Study the drawing (mm; zero at the part's minimum x, y, z) and answer. Round coordinates to 2 decimals unless told otherwise and drop trailing zeros. Loops run counter-clockwise (first coordinate to the right, second up) from the corner with the lowest first, then second, coordinate; pieces in that order, holes last. Notation, with made-up numbers: M -27,-14 L 6,-14 A13 cw 6,-10 Z; hole C -1,-32 d7. An arc over 180 degrees is marked long. Write each question's results on one line, items separated by ' | '.
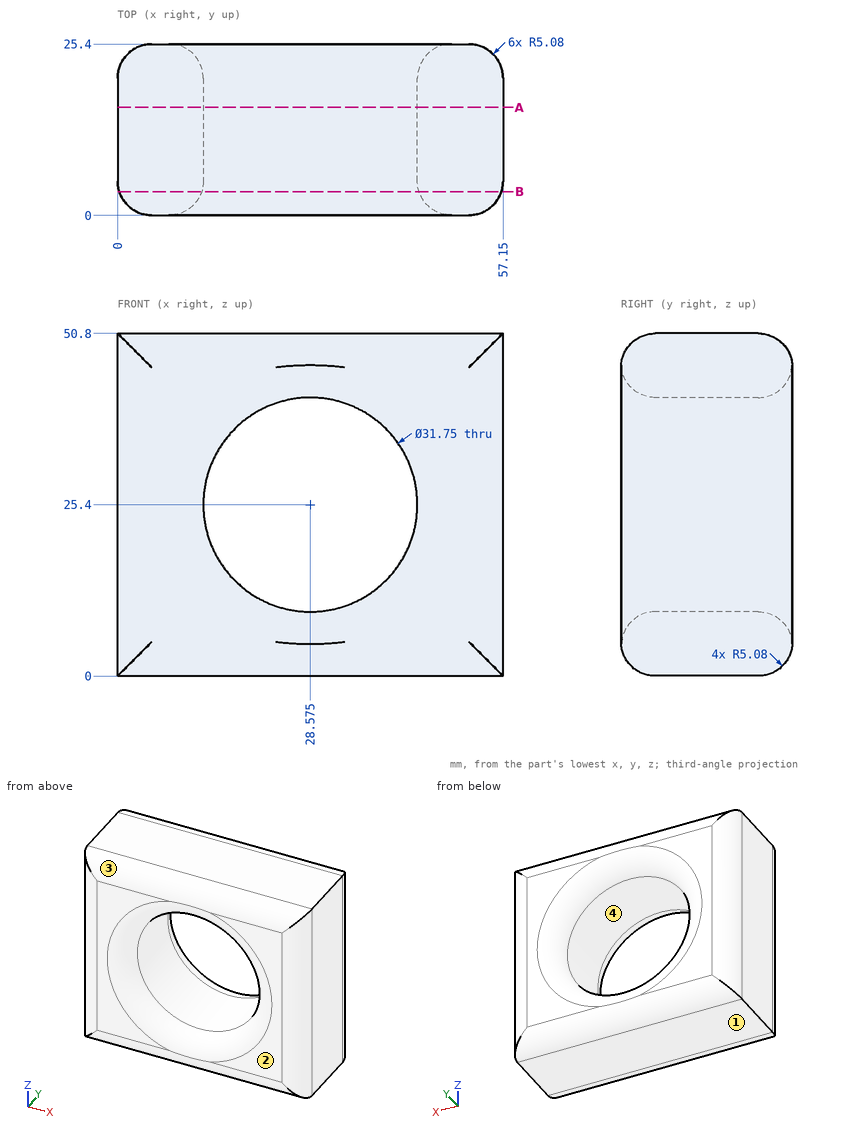
Item 1: The part is cut by section B-B (y = 3.5). Determine the outline of the cut face in (x, z) (3 decimals).
Outcome:
outline: M 0.252,0.252 L 56.898,0.252 L 56.898,50.548 L 0.252,50.548 Z; hole C 28.575,25.4 d32.254
Item 2: Straight lines are drawn through the part: line 1 (X direction, y = 13.25, z = 25); line 2 (Y direction, x = 5, z = 22.5); line 3 (Z direction, x = 14, y = 8). For each, find the intervals that lie inside material, in ascending order.
Outcome:
line 1: x = 0 to 12.71, 44.44 to 57.15 | line 2: y = 0 to 25.4 | line 3: z = 0 to 19.11, 31.69 to 50.8
Item 3: The part is cut by section A-A (y = 16). Determine the outline of the cut face in (x, z) (3 decimals).
Outcome:
outline: M 0,0 L 57.15,0 L 57.15,50.8 L 0,50.8 Z; hole C 28.575,25.4 d31.75
Item 4: Flat-ended cylindrical pins translate along their axes: pin 1 (8 mm diameter, centred on y = 20.5, z = 43.5, fed in from -X); pin 2 (8 mm diameter, centred on x = 37.5, z = 37, fed in from +Y); pin 3 (2 mm diameter, centred on x = 31.5, y = 21.5, fed in from -Z). Find the tip coordinate at first contact, or state that the pin passes through.
Outcome:
pin 1: stops at x = 0 | pin 2: stops at y = 24.84 | pin 3: stops at z = 0
Item 5: The mould has two halves that part along Z. Classify the marked faces 1, 2, 3 and 4: pulls with the +Z half, pulls with the -Z half, needs draft (parallel to the pull), parting line crosses it, or undercut.
Outcome:
face 1: pulls with the -Z half | face 2: needs draft | face 3: pulls with the +Z half | face 4: undercut
